Design review of the part built by this model. Coordinates are the model's own, in mm. A direction names the side the tool comes from. Coordinates: 2 decimals unless noted, no trailing zeros. Write each loop counter-clockwise with the first axis right and the second up, starting at its lowest first coordinate (ties: lowest second). Pieces come first, ordered by that corner, then holes. Notation, with made-up numbers: (88.25, -34) - (95.25, -34) arc R19 ccw to (95.25, 1) - close; hole circle Ø1 at (70.25, -38). An arc over 180 degrees is marked (long way). Use a Markdown table: item, result.
from build123d import *

# Parameters (mm, degrees)
SKETCH_W        = 190
SKETCH_H        = 190
SKETCH_W_2      = 160
SKETCH_H_2      = 160
PAD_DEPTH       = 20
SKETCH001_R     = 1.5
SKETCH001_R_2   = 2
POCKET_DEPTH    = 20.001
SKETCH002_R     = 4
POCKET001_DEPTH = 15
POCKET002_DEPTH = 13
CHAMFER_SIZE    = 1


with BuildPart() as part:
    # Sketch → Pad (new body)
    with BuildSketch(Plane.XY):
        with Locations((95, 95)):
            Rectangle(SKETCH_W, SKETCH_H)
        with Locations((95, 95)):
            Rectangle(SKETCH_W_2, SKETCH_H_2, mode=Mode.SUBTRACT)
    extrude(amount=-PAD_DEPTH)

    # Sketch001 → Pocket (cut, through all)
    with BuildSketch(Plane.XY):
        with Locations((10, 22)):
            Circle(SKETCH001_R)
        with Locations((10, 107.5)):
            Circle(SKETCH001_R)
        with Locations((10, 168)):
            Circle(SKETCH001_R)
        with Locations((107.5, 180)):
            Circle(SKETCH001_R)
        with Locations((180, 168)):
            Circle(SKETCH001_R)
        with Locations((180, 82.5)):
            Circle(SKETCH001_R)
        with Locations((180, 22)):
            Circle(SKETCH001_R)
        with Locations((82.5, 10)):
            Circle(SKETCH001_R)
        with Locations((33, 183)):
            Circle(SKETCH001_R_2)
        with Locations((157, 7)):
            Circle(SKETCH001_R_2)
    extrude(amount=-POCKET_DEPTH, mode=Mode.SUBTRACT)

    # Sketch002 → Pocket001 (cut)
    with BuildSketch(Plane.XY):
        with Locations((107.5, 180)):
            Circle(SKETCH002_R)
        with Locations((180, 168)):
            Circle(SKETCH002_R)
        with Locations((10, 168)):
            Circle(SKETCH002_R)
        with Locations((10, 107.5)):
            Circle(SKETCH002_R)
        with Locations((10, 22)):
            Circle(SKETCH002_R)
        with Locations((82.5, 10)):
            Circle(SKETCH002_R)
        with Locations((180, 22)):
            Circle(SKETCH002_R)
        with Locations((180, 82.5)):
            Circle(SKETCH002_R)
    extrude(amount=-POCKET001_DEPTH, mode=Mode.SUBTRACT)

    # Sketch003 → Pocket002 (cut)
    with BuildSketch(Plane.XY):
        Polygon((90, 0), (100, 0), (100, 10), (101.5, 15), (88.5, 15), (90, 10), align=None)
    extrude(amount=-POCKET002_DEPTH, mode=Mode.SUBTRACT)

    # Chamfer
    chamfer_edges = [part.edges().sort_by_distance(p)[0] for p in [
        (0, 95, 0),
        (45, 0, 0),
        (145, 0, 0),
        (190, 95, 0),
        (95, 190, 0),
        (100, 5, 0),
        (90, 5, 0),
    ]]
    chamfer(chamfer_edges, length=CHAMFER_SIZE)


solid = part.part
(1) Machinability: for faces 1 (the cylindrical face through (6.004, 107.676, -7.395)), 2 (the flat face through (15, 94, -10)), 3 (the flat face through (94, 180, 0)), which of the approach directions +Z, -Z, +X, -X, +Y, -Y give a long, thin tool a straight path to every point of the face, cutting with its end or side? Answer none if there is none.
Determined:
| item | result |
|---|---|
| face 1 | +Z |
| face 2 | +Z, -Z |
| face 3 | +Z, +X, -X, +Y, -Y |
(2) For L1, parallel to Y at x = 10, z = -16.4; L2, parallel to X at y = 168, z = -17.65; L3, parallel to Y at x = 180, z = -18.1, list the stretches that pass through material, from the lowest coordinate up. Write a range as from..to.
Determined:
| item | result |
|---|---|
| L1 | 0..20.5, 23.5..106, 109..166.5, 169.5..190 |
| L2 | 0..8.5, 11.5..15, 175..178.5, 181.5..190 |
| L3 | 0..20.5, 23.5..81, 84..166.5, 169.5..190 |
(3) Draft analysis for pull direction Y (two halves, no side actions). For faces 4 (the flat face through (94, 15, -14)), 5 (the flat face through (0, 94, -10)), 6 (the flat face through (94, 190, -10)), state which applies: +Y half, -Y half, draft (parallel to the pull), parting line (faces both ways), or undercut.
Determined:
| item | result |
|---|---|
| face 4 | undercut |
| face 5 | draft |
| face 6 | +Y half |
(4) Take a section at A-A on x = 162. Write out the cut boundary in (y, z).
Determined:
| item | result |
|---|---|
| outline | (0, -20) - (15, -20) - (15, 0) - (1, 0) - (0, -1) - close; (175, -20) - (190, -20) - (190, -1) - (189, 0) - (175, 0) - close |
(5) For pin 1 (2.5 mm diameter, centred on x = 10, y = 22, fed in from +Z); pin 2 (3.5 mm diameter, centred on x = 180, y = 82.5, fed in from +Z); pin 3 (4 mm diameter, centred on x = 92.5, y = 6.5, fed in from +Z), all flat-tipped, find the tip position at first contact; note any pin that passes through.
Determined:
| item | result |
|---|---|
| pin 1 | through |
| pin 2 | z = -15 |
| pin 3 | z = -13 |
